Autodesk Inventor part; units mm, degrees
ref_plane "YZ Plane" through (0, 0, 0) normal (1, 0, 0) x (0, 1, 0)
ref_plane "XZ Plane" through (0, 0, 0) normal (0, 1, 0) x (-1, 0, 0)
ref_plane "XY Plane" through (0, 0, 0) normal (0, 0, 1) x (1, 0, 0)
sketch "Sketch1" plane through (0, 0, 0) normal (0, 0, 1) x (1, 0, 0)
  line L0 (-75, 25) -> (75, 25)
  line L1 (75, 25) -> (75, -25)
  line L2 (75, -25) -> (-75, -25)
  line L3 (-75, -25) -> (-75, 25)
  line L4 (-75, 25) -> (75, -25) construction
  line L5 (75, 25) -> (-75, -25) construction
  line L6 (25, 25) -> (25, -25)
  line L7 (22.5, 25) -> (27.5, 25)
  line L8 (27.5, 25) -> (27.5, -25)
  line L9 (27.5, -25) -> (22.5, -25)
  line L10 (22.5, -25) -> (22.5, 25)
  line L11 (22.5, 25) -> (27.5, -25) construction
  line L12 (27.5, 25) -> (22.5, -25) construction
  line L13 (75, 25) -> (70, 25)
  line L14 (70, 25) -> (70, -25)
  line L15 (70, -25) -> (75, -25)
  line L16 (75, -25) -> (75, 25)
  point P0 (0, 0)
  point P1 (25, 0)
  point P2 (22.5, 25)
  point P3 (22.5, -25)
  point P4 (27.5, -25)
  point P5 (27.5, 25)
  dimension "d0" = 50
  dimension "d1" = 150
  dimension "d9" = 50
  dimension "d14" = 5
  dimension "d15" = 5
sketch "Sketch2" plane through (0, 0, 0) normal (1, 0, 0) x (0, 1, 0)
  line L0 (25, 0) -> (-25, 0)
  line L1 (25, 0) -> (-25, 0)
  line L2 (-25, 0) -> (-25, 70)
  line L3 (-25, 70) -> (25, 70)
  line L4 (25, 70) -> (25, 0)
  line L5 (-20, 70) -> (5.4779, 0)
  line L6 (25, 5) -> (-25, 5)
  line L7 (-20, 70) -> (-20, 0)
  point P0 (0, 0)
  point P1 (5.4779, 0)
  point P2 (3.6581, 5)
  dimension "d2" = 70
  dimension "d3" = 5
  dimension "d5" = 5
  dimension "d20" = 20
extrude "Extrusion1" add sketch "Sketch2" along normal blind 75 contours L0 L7 L6 L5 | L0 L2 L6 L7 | L6 L7 L5 | L6 L2 L3 L7
extrude "Extrusion2" add sketch "Sketch2" along normal blind 75 contours L0 L5 L6 L4
extrude "Extrusion3" add sketch "Sketch1" along normal blind 70 contours L0 L1 L2 L14
extrude "Extrusion4" add sketch "Sketch1" along normal blind 70 contours L0 L6 L2 L10 | L0 L8 L2 L6
mirror "Mirror1" about plane through (0, 0, 0) normal (1, 0, 0)
fillet "Fillet1" radius 2 9 edges at (-27.5, 25, 37.5) (-22.5, 25, 37.5) (22.5, 25, 37.5) (27.5, 25, 37.5) (70, 25, 37.5) (-70, 25, 37.5) (-48.75, 25, 5) (0, 25, 5) (48.75, 25, 5)
fillet "Fillet2" radius 2 10 edges at (-25, 25, 70) (-22.5, 1.5, 70) (-27.5, 1.5, 70) (25, 25, 70) (27.5, 1.5, 70) (22.5, 1.5, 70) (73.5, 25, 70) (70, 1.5, 70) (-73.5, 25, 70) (-70, 1.5, 70)
sketch "Sketch3" plane through (75, -25, 0) normal (0, -1, 0) x (1, 0, 0)
  line L0 (0, 0) -> (-150, 0)
  line L1 (0, 70) -> (0, 0)
  line L2 (-150, 70) -> (0, 70)
  line L3 (-150, 70) -> (-150, 0)
  line L4 (-145, 5) -> (-5, 5)
  line L5 (-5, 5) -> (-5, 65)
  line L6 (-5, 65) -> (-145, 65)
  line L7 (-145, 65) -> (-145, 5)
  circle A0 centre (-5, 5) radius 2.7
  circle A1 centre (-145, 5) radius 2.75
  point P0 (-75, 0)
  dimension "d35" = 5
  dimension "d36" = 5.4
  dimension "d37" = 5.5
extrude "Extrusion5" cut sketch "Sketch3" against normal blind 10 contours L7 A1 L4 | L4 A1 L7 | A0 L5 L4 | L4 L5 A0
fillet "Fillet3" radius 1 2 edges at (67.3, -25, 5) (-72.75, -25, 5)
ref_plane "Work Plane2" through (75, -25, 5) normal (0, 0, -1) x (-1, 0, 0)
fillet "Fillet4" radius 1 1 edges at (-72.75, -15, 5)
fillet "Fillet5" radius 1 1 edges at (67.3, -15, 5)
equation "\"d9\" = 0.333333 * d1"
equation "\"d5\" = d3"
equation "\"d10\" = 0.5 * d1"
equation "\"d12\" = 0.5 * d1"
equation "\"d16\" = d2"
equation "\"d18\" = d2"
properties part number "rubbish-container-group2" material "ABS Plastic"
Here's how the part is built. I have some questions about the finished solid (model axes, mm). A direction names the side the tool comes from. Round coordinates to 2 decimals unless told otherwise and drop trailing zeros. Loops run counter-clockwise (first coordinate to the right, second up) from the corner with the lowest first, then second, coordinate; pieces in that order, holes last.
1. If we section it at C-C on z = 60: Write out the boundary of the cut face in (x, y).
Answer list:
outline: (-75, -25) - (75, -25) - (75, 25) - (72, 25) arc R2 ccw to (70, 23) - (70, -16.36) - (27.5, -16.36) - (27.5, 23) arc R2 ccw to (25.5, 25) - (24.5, 25) arc R2 ccw to (22.5, 23) - (22.5, -16.36) - (-22.5, -16.36) - (-22.5, 23) arc R2 ccw to (-24.5, 25) - (-25.5, 25) arc R2 ccw to (-27.5, 23) - (-27.5, -16.36) - (-70, -16.36) - (-70, 23) arc R2 ccw to (-72, 25) - (-75, 25) - close
2. Which directions (+Z, -Z, +X, -X, +Y, -Y) give clear straight access to the entire face, cutting with the end or side of a thin tool? Please do faces 1 (the face through (70, -15, 5)), 2 (the face through (70, 7, 43)), 3 (the face through (-75, 0, 35)).
Answer list:
face 1: -Y
face 2: +Z, +Y
face 3: +Z, -Z, -X, +Y, -Y
3. If I drill on line 1 along X through (y, z) = (15, 65.5); line 2 along X through (y, z) = (-20.25, 5); line 3 along Z through (x, y) = (-70, -20.5), over which ranges is the centre line in solid material (lowest first)?
Answer list:
line 1: x = -75 to -70, -27.5 to -22.5, 22.5 to 27.5, 70 to 75
line 2: x = -75 to -72.75, -67.25 to 67.3, 72.7 to 75
line 3: z = 0 to 2.25, 7.75 to 70
4. If we section it at B-B on x = -38: Write out the boundary of the cut face in (y, z).
Answer list:
outline: (-25, 0) - (25, 0) - (25, 3) arc R2 ccw to (23, 5) - (3.66, 5) - (-20, 70) - (-25, 70) - close
5. For P1, Ø4.5, axis at x = -70, z = 5, coming from the -Y side; P2, Ø21.5, axis at x = -44.5, y = 14.5, coming from the +Z side; P3, Ø3.5, axis at x = 69.5, z = 5.5, coming from the -Y side, each with a flat end and sliding along its axis, tell me the tip position at first contact or that it passes through.
Answer list:
P1: stops at y = -15.13
P2: stops at z = 5
P3: stops at y = -15.35
6. If we section it at A-A on y = 21: Write out the boundary of the cut face in (x, z).
Answer list:
outline: (-75, 0) - (75, 0) - (75, 70) - (72, 70) arc R2 ccw to (70, 68) - (70, 5) - (27.5, 5) - (27.5, 68) arc R2 ccw to (25.5, 70) - (24.5, 70) arc R2 ccw to (22.5, 68) - (22.5, 5) - (-22.5, 5) - (-22.5, 68) arc R2 ccw to (-24.5, 70) - (-25.5, 70) arc R2 ccw to (-27.5, 68) - (-27.5, 5) - (-70, 5) - (-70, 68) arc R2 ccw to (-72, 70) - (-75, 70) - close
